```python
from build123d import *

# Parameters (mm, degrees)
F3_DEPTH        = 4
F5_DEPTH        = 4
F7_DEPTH        = 4
F8_DEPTH        = 2
F8_COPIES_COUNT = 3
F10_W           = 40
F10_H           = 6
F11_DEPTH       = 25
F11_DEPTH_BACK  = 25
F12_R           = 3


# Not quite as in the source:
# - an extrude whose draft closes it to a point is written as a loft to that point
# - a feature of the source that left no trace in its solid (it failed there, or was rolled back) is left out
# - a pattern or mirror of a feature is missing from the dataset's text; its kind, count and spacing are read off the source's solid


with BuildPart() as f0:
    # F13 (on Top) → F0 section 0
    with BuildSketch(Plane.XY, mode=Mode.PRIVATE) as f0_s0:
        Polygon((-21.5980762114, -12.4696551146), (21.5980762114, -12.4696551146), (0, 24.9393102292), align=None)
    loft([f0_s0.sketch, Vertex(0, 0, 64.1508142976)], ruled=True)

    # F1 (on face) → F3 (cut)
    with BuildSketch(Plane(origin=(0, -12.0156590044, 2.3356075118), x_dir=(1, 0, 0), z_dir=(0, -0.9816271834, 0.1908089954))):
        Polygon((-4.8375685578, 27.6206776349), (-14.7522947938, -2.3793223651), (0, -2.3793223651), (14.7522947938, -2.3793223651), (4.8375685578, 27.6206776349), (1.25, 27.6206776349), (1.25, 22.6206776349), (0, 22.6206776349), (-1.25, 22.6206776349), (-1.25, 27.6206776349), align=None)
    extrude(amount=-F3_DEPTH, mode=Mode.SUBTRACT)

    # F4 (on face) → F5 (cut)
    with BuildSketch(Plane(origin=(10.4058659411, 6.0078295022, 2.3356075118), x_dir=(-0.4788987638, 0.8712646086, -0.1074893292), z_dir=(0.8501140779, 0.4908135917, 0.1908089954))):
        Polygon((-7.8329752774, 26.9248658467), (-14.40304573, -3.980408308), (0.2605385928, -2.3650147058), (14.9241229157, -0.7496211036), (1.7839820104, 27.9843047215), (-1.7820133006, 27.5914617519), (-1.2345074295, 22.6215284202), (-2.4769907625, 22.4846519525), (-3.7194740954, 22.3477754847), (-4.2669799664, 27.3177088164), align=None)
    extrude(amount=-F5_DEPTH, mode=Mode.SUBTRACT)

    # F6 (on face) → F7 (cut)
    with BuildSketch(Plane(origin=(-10.4058659411, 6.0078295022, 2.3356075118), x_dir=(-0.4788987638, -0.8712646086, 0.1074893292), z_dir=(-0.8501140779, 0.4908135917, 0.1908089954))):
        Polygon((-1.7839820104, 27.9843047215), (-14.9241229157, -0.7496211036), (-0.2605385928, -2.3650147058), (14.40304573, -3.980408308), (7.8329752774, 26.9248658467), (4.2669799664, 27.3177088164), (3.7194740954, 22.3477754847), (2.4769907625, 22.4846519525), (1.2345074295, 22.6215284202), (1.7820133006, 27.5914617519), align=None)
    extrude(amount=-F7_DEPTH, mode=Mode.SUBTRACT)

    # F1 (on face) → F8 (join)
    with BuildSketch(Plane(origin=(0, -12.0156590044, 2.3356075118), x_dir=(1, 0, 0), z_dir=(0, -0.9816271834, 0.1908089954))):
        Polygon((-4.8375685578, 27.6206776349), (-14.7522947938, -2.3793223651), (0, -2.3793223651), (14.7522947938, -2.3793223651), (4.8375685578, 27.6206776349), (1.25, 27.6206776349), (1.25, 22.6206776349), (0, 22.6206776349), (-1.25, 22.6206776349), (-1.25, 27.6206776349), align=None)
    f8 = extrude(amount=-F8_DEPTH)

    # F8_copies: F8 ×3 about axis
    f8_copies_axis = Axis((0, 0, 0), (0, 0, 1))
    for i in range(1, F8_COPIES_COUNT):
        add(f8.rotate(f8_copies_axis, i * 360 / F8_COPIES_COUNT))

    # F10 (on Right) → F11 (cut, two sides)
    with BuildSketch(Plane.YZ) as f11_sk:
        with Locations((6, 2)):
            Rectangle(F10_W, F10_H)
    extrude(amount=-F11_DEPTH, mode=Mode.SUBTRACT)
    extrude(f11_sk.sketch, amount=F11_DEPTH_BACK, mode=Mode.SUBTRACT)

    # F12
    f12_edges = [f0.edges().sort_by_distance(p)[0] for p in [
        (-9.957347, -5.748877, 34.575407),
        (9.957347, -5.748877, 34.575407),
        (0, 11.497754, 34.575407),
    ]]
    fillet(f12_edges, radius=F12_R)


solid = f0.part
```
Part model, mm, in its own coordinate system. Round coordinates to 2 decimals unless told otherwise and drop trailing zeros. Use one line per item in the form item = value. Start each with the question number.
Item 1: Band-saw the part on A-A (z = 19). Give the number of separate pieces and of enclosed holes in the cut face, plus the area to 3 significant figures.
Item 2: Drill centre lines: line 1 along Y through (x, z) = (-5, 8.5); line 2 along Y through (x, z) = (6, 21.5); line 3 along X through (y, z) = (12.5, 13.5). Where is each one in solid material? Low to high.
Item 3: Drop flat-ended pins along their axis: pin 1 Ø3 at (x, z) = (13, 15) entering from -Y; pin 2 Ø10 at (y, z) = (-6.5, 26.5) entering from +X; pin 3 Ø12 at (x, z) = (-10, 33) entering from -Y. Give the stop position or say it passes through.
Item 4: Two-plate mould, pull along Z, no slides. Class faces 1 (the flat face through (3.086, 3.225, 26.459)), 2 (the flat face through (0, -3, 5)): released by +Z, released by -Z, zero draft, split by the parting line, or undercut.
Data:
q1.separate_pieces = 1
q1.enclosed_holes = 3
q1.area = 283 mm^2
q2.line_1 = -10.82 to -8.78, -6.74 to 4.82, 8.9 to 12.97
q2.line_2 = -8.29 to -6.25, -4.22 to -1.96, 2.11 to 6.19
q2.line_3 = -4.15 to -1.8, -1.52 to 1.52, 1.8 to 4.15
q3.pin_1 = -9.79
q3.pin_2 = 12.2
q3.pin_3 = -7.1
q4.face_1 = undercut
q4.face_2 = released by -Z
